```python
from build123d import *

# Parameters (mm, degrees)
SKETCH1_W       = 12.7
SKETCH1_H       = 12.7
EXTRUDE1_DEPTH  = 8.255
SKETCH2_R       = 4
EXTRUDE2_DEPTH  = 12.7
SKETCH4_R       = 4
EXTRUDE8_DEPTH  = 2.5
EXTRUDE8_TAPER  = 51
SKETCH5_R       = 0.25
EXTRUDE9_DEPTH  = 2.5
SKETCH3_R       = 1.75
EXTRUDE10_DEPTH = 20.955
SKETCH7_R       = 2.5
EXTRUDE11_DEPTH = 12.7
SKETCH8_R       = 0.5
EXTRUDE12_DEPTH = 2.5


with BuildPart() as part:
    # Sketch1 → Extrude1 (new body)
    with BuildSketch(Plane(origin=(0, 0, 0), x_dir=(1, 0, 0), z_dir=(0, 1, 0))):
        Rectangle(SKETCH1_W, SKETCH1_H)
    extrude(amount=EXTRUDE1_DEPTH)

    # Sketch2 → Extrude2 (add)
    with BuildSketch(Plane(origin=(0, 8.255, 0), x_dir=(1, 0, 0), z_dir=(0, 1, 0))):
        with Locations((0, -1.85)):
            Circle(SKETCH2_R)
    extrude(amount=EXTRUDE2_DEPTH)

    # Sketch4 → Extrude8 (add)
    with BuildSketch(Plane.XZ):
        with Locations((0, 1.85)):
            Circle(SKETCH4_R)
    extrude(amount=EXTRUDE8_DEPTH, taper=EXTRUDE8_TAPER)

    # Sketch5 → Extrude9 (cut)
    with BuildSketch(Plane.XZ.offset(2.5)):
        with Locations((0, 1.85)):
            Circle(SKETCH5_R)
    extrude(amount=-EXTRUDE9_DEPTH, mode=Mode.SUBTRACT)

    # Sketch3 → Extrude10 (cut)
    with BuildSketch(Plane(origin=(0, 20.955, 0), x_dir=(-1, 0, 0), z_dir=(0, 1, 0))):
        with Locations((0, 1.85)):
            Circle(SKETCH3_R)
    extrude(amount=-EXTRUDE10_DEPTH, mode=Mode.SUBTRACT)

    # Sketch7 → Extrude11 (cut)
    with BuildSketch(Plane.ZY.offset(6.35)):
        with Locations((-2.85, 4.1275)):
            Circle(SKETCH7_R)
    extrude(amount=-EXTRUDE11_DEPTH, mode=Mode.SUBTRACT)

    # Sketch8 → Extrude12 (cut)
    with BuildSketch(Plane.XY.offset(6.35)):
        with Locations((-4.199914645, 2.150085355)):
            Circle(SKETCH8_R)
    extrude(amount=-EXTRUDE12_DEPTH, mode=Mode.SUBTRACT)


solid = part.part
```
Verification items for the finished model (mm, model axes). A direction names the side the tool comes from. Coordinates: 2 decimals unless noted, no trailing zeros. Loops run counter-clockwise (first coordinate to the right, second up) from the corner with the lowest first, then second, coordinate; pieces in that order, holes last. Notation, with made-up numbers: (29, 75.25) -> (37, 75.25) arc R20 cw to (37, 109.25) -> close; hole circle Ø9 at (39, -11.75). An arc over 180 degrees is marked (long way). Answer in a Markdown table with one row per item. Add a question column.
1. Material ranges on probe 1 along Y at (x, z) = (-2.5, -2.85) (1 decimal); probe 2 along Z at (x, y) = (0, 10); probe 3 along Y at (x, z) = (3, 4.75) (3 decimals), recorded low to high. Write a range as [from, to].
2. Section check B-B, the plane y = 3.5. Enter the section's corners in (x, z), then the cut area to 3 significant figures.
3. Draft check along X on faces 4 (the face through (-6.35, 4, 0)), 5 (the face through (-4, 2, 3.85)), 6 (the face through (-0.81, 10.62, 0.3)), 7 (the face through (-0.089, 4.237, -5.348)). Enter one of: +X half, -X half, draft (parallel to the pull), parting line (faces both ways), or undercut.
4. Section check D-D, the plane y = 7.5. Enter the section's corners in (x, z), then the cut area to 3 significant figures.
5. Access from +Z, -Z, +X, -X, +Y, -Y to the whole of each face (thin tool, end or side, straight path). Record for faces 1 (the face through (3.8, 14.5, 0.6)), 2 (the face through (6.35, 4, 0)), 3 (the face through (-3.723, 2.3, 5.118)).
6. Section check C-C, the plane x = 0. Give the number of separate pieces and of enclosed holes in the cut face, then the cut area to 3 significant figures.
7. Depth check by flat-ended pin: P1, Ø5, axis at y = 16, z = -0.5, coming from the -X side. Enter the tip coordinate at first touch or a pass-through.
Derived:
| question | item | result |
|---|---|---|
| 1 | probe 1 | y = [0, 1.6], [6.6, 8.3] |
| 1 | probe 2 | z = [-2.15, 0.1], [3.6, 5.85] |
| 1 | probe 3 | y = [0, 8.255] |
| 2 | outline | (-6.35, -6.35) -> (6.35, -6.35) -> (6.35, -5.27) -> (-6.35, -5.27) -> close; (-6.35, -0.43) -> (6.35, -0.43) -> (6.35, 6.35) -> (-6.35, 6.35) -> close; hole circle Ø3.5 at (0, 1.85) |
| 2 | area | 90.2 mm² |
| 3 | face 4 | -X half |
| 3 | face 5 | undercut |
| 3 | face 6 | undercut |
| 3 | face 7 | draft |
| 4 | outline | (-6.35, -6.35) -> (6.35, -6.35) -> (6.35, 6.35) -> (-6.35, 6.35) -> close; hole circle Ø3.5 at (0, 1.85) |
| 4 | area | 152 mm² |
| 5 | face 1 | +Y |
| 5 | face 2 | +Z, -Z, +X, +Y, -Y |
| 5 | face 3 | +Z |
| 6 | separate pieces | 2 |
| 6 | enclosed holes | 1 |
| 6 | area | 124 mm² |
| 7 | P1 | stops at x = -4 |
